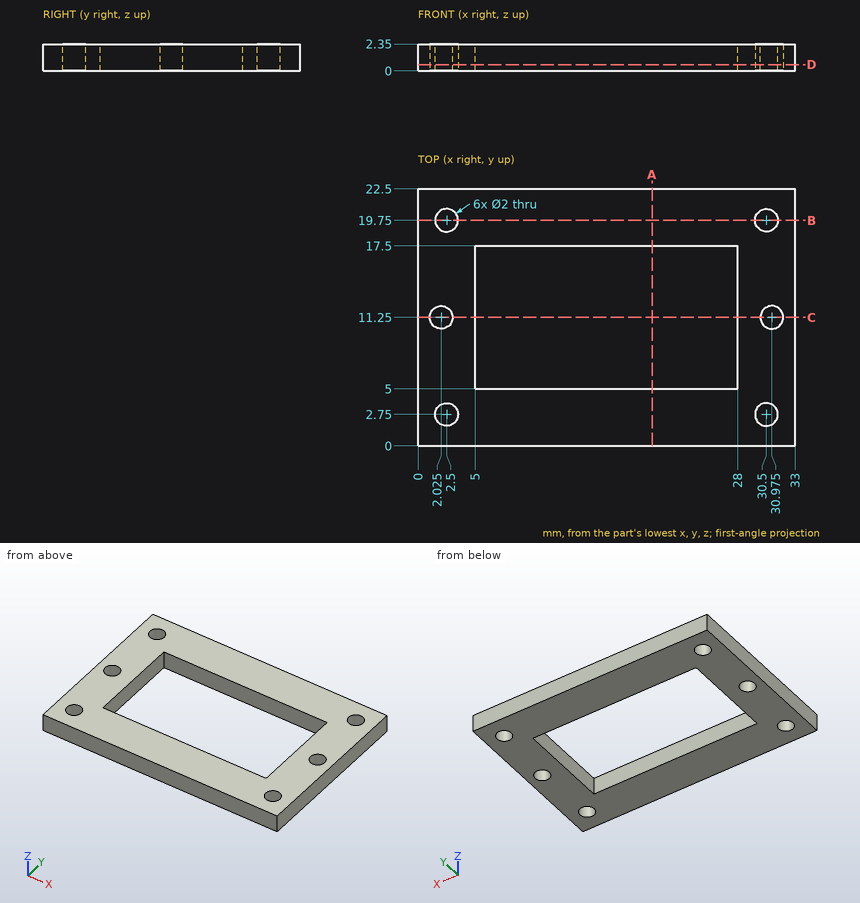
Check sheet for the drawn part. Datum: minimum x, y, z corner. Units: mm. Coordinates: 2 decimals unless noted, no trailing zeros. Write each loop counter-clockwise with the first axis right and the second up, starting at its lowest first coordinate (ties: lowest second). Pieces come first, ordered by that corner, then holes. Notation, with made-up numbers: M 1,-24.75 L 51,-24.75 A7 cw 51,-17.75 Z; hole C 79,37 d2. An arc over 180 degrees is marked long. Use a Markdown table: item, result.
Q1. Sectioned sample at B-B, the plane y = 19.75. Record the boundary of the cut face in (x, z).
Reply:
| item | result |
|---|---|
| outline | M 0,0 L 1.5,0 L 1.5,2.35 L 0,2.35 Z; M 3.5,0 L 29.5,0 L 29.5,2.35 L 3.5,2.35 Z; M 31.5,0 L 33,0 L 33,2.35 L 31.5,2.35 Z |
Q2. Sectioned sample at C-C, the plane y = 11.25. Record the boundary of the cut face in (x, z) (3 decimals).
Reply:
| item | result |
|---|---|
| outline | M 0,0 L 1.025,0 L 1.025,2.35 L 0,2.35 Z; M 3.025,0 L 5,0 L 5,2.35 L 3.025,2.35 Z; M 28,0 L 29.975,0 L 29.975,2.35 L 28,2.35 Z; M 31.975,0 L 33,0 L 33,2.35 L 31.975,2.35 Z |
Q3. Sectioned sample at D-D, the plane z = 0.55. Record the boundary of the cut face in (x, y) (3 decimals), plus the area to 3 significant figures.
Reply:
| item | result |
|---|---|
| outline | M 0,0 L 33,0 L 33,22.5 L 0,22.5 Z; hole C 2.025,11.25 d2; hole C 2.5,2.75 d2; hole C 2.5,19.75 d2; hole M 5,5 L 28,5 L 28,17.5 L 5,17.5 Z; hole C 30.5,2.75 d2; hole C 30.5,19.75 d2; hole C 30.975,11.25 d2 |
| area | 436 mm² |
Q4. Sectioned sample at A-A, the plane x = 20.5. Record the boundary of the cut face in (y, z), plus the area to 3 significant figures.
Reply:
| item | result |
|---|---|
| outline | M 0,0 L 5,0 L 5,2.35 L 0,2.35 Z; M 17.5,0 L 22.5,0 L 22.5,2.35 L 17.5,2.35 Z |
| area | 23.5 mm² |
Q5. Thickness scan on line 1 (Y direction, x = 26, z = 1.1); line 2 (X direction, y = 2.75, z = 0.6); line 3 (X direction, y = 16.5, z = 0.7). Record the ranges inside material, lowest first.
Reply:
| item | result |
|---|---|
| line 1 | y = 0 to 5, 17.5 to 22.5 |
| line 2 | x = 0 to 1.5, 3.5 to 29.5, 31.5 to 33 |
| line 3 | x = 0 to 5, 28 to 33 |
